Source: CAD feature listing. Evaluate the final solid. Frame: model axes, mm. A direction names the side the tool comes from. Give positions to 0.01 mm unless a question says otherwise; leave off trailing zeros. Order: outer loops, then holes, each group sorted by start corner. A loop starts at its lowest first (then second) coordinate and runs counter-clockwise, first axis right, second up. Notation, with made-up numbers: (28.25, -31) -> (66.25, -31) arc R30 ccw to (66.25, -3) -> close; hole circle Ø11 at (61.5, -23). An arc over 180 degrees is marked (long way). Use CSV: the item, a comma, the result in double quotes.
```python
from build123d import *

# Parameters (mm, degrees)
SKETCH_1_W           = 16
SKETCH_1_H           = 11
EXTRUDE_1_DEPTH      = 25
SKETCH_2_OUTSIDE_W   = 215.706
SKETCH_2_OUTSIDE_H   = 63.306
SKETCH_2_OUTSIDE_R   = 2.15
SKETCH_2_OUTSIDE_R_2 = 6.85
CUT_EXTRUDE_1_DEPTH  = 182.533054841
SKETCH_3_R           = 7.8
CUT_EXTRUDE_2_DEPTH  = 1.3
SKETCH_4_R           = 7.85
CUT_EXTRUDE_3_DEPTH  = 1.3
CUT_EXTRUDE_5_DEPTH  = 7
SKETCH_5_3_R         = 1.50558517
CUT_EXTRUDE_6_DEPTH  = 181.299334441


with BuildPart() as part:
    # 草图1 → 凸台-拉伸1 (new body)
    with BuildSketch(Plane(origin=(0, 0, 0), x_dir=(1, 0, 0), z_dir=(0, 1, 0))):
        Polygon((0, 0), (0, 19), (127, 19), (161, 20.3), (177.4, 20.3), (177.4, 13.4), (146, 13.4), (146, -2.1), (177.4, -2.1), (177.4, -9), (144, -9), (127, 0), align=None)
        with Locations((39, 9.5)):
            Rectangle(SKETCH_1_W, SKETCH_1_H, mode=Mode.SUBTRACT)
        Polygon((126, 15), (126, 4), (143, -5), (143, 15.65), align=None, mode=Mode.SUBTRACT)
        with Locations((58, 9.5)):
            Rectangle(SKETCH_1_W, SKETCH_1_H, mode=Mode.SUBTRACT)
        with Locations((77, 9.5)):
            Rectangle(SKETCH_1_W, SKETCH_1_H, mode=Mode.SUBTRACT)
        with Locations((96, 9.5)):
            Rectangle(SKETCH_1_W, SKETCH_1_H, mode=Mode.SUBTRACT)
        with Locations((115, 9.5)):
            Rectangle(SKETCH_1_W, SKETCH_1_H, mode=Mode.SUBTRACT)
    extrude(amount=EXTRUDE_1_DEPTH)

    # 草图2 outside → 切除-拉伸1 (cut, through all)
    # profile 1 of 3: a face of its own
    with BuildSketch(Plane.XY.offset(9)):
        with Locations((88.7, 12.5)):
            Rectangle(SKETCH_2_OUTSIDE_W, SKETCH_2_OUTSIDE_H)
        Polygon((0, 21.701223904), (3.298776096, 25), (172.796734854, 16.606530291), (177.4, 12.003265146), (177.4, 4.603265146), (172.796734854, 0), (4.701223904, 0), (0, 4.701223904), align=None, mode=Mode.SUBTRACT)
    # profile 2 of 3: a face of its own
    with BuildSketch(Plane.XY.offset(9)):
        with Locations((169.9, 8.303265146)):
            Circle(SKETCH_2_OUTSIDE_R)
    # profile 3 of 3: a face of its own
    with BuildSketch(Plane.XY.offset(9)):
        with Locations((12, 13.201223904)):
            Circle(SKETCH_2_OUTSIDE_R_2)
    extrude(amount=-CUT_EXTRUDE_1_DEPTH, mode=Mode.SUBTRACT)

    # 草图3 → 切除-拉伸2 (cut)
    with BuildSketch(Plane.XY):
        with Locations((12, 13.201223904)):
            Circle(SKETCH_3_R)
    extrude(amount=-CUT_EXTRUDE_2_DEPTH, mode=Mode.SUBTRACT)

    # 草图4 → 切除-拉伸3 (cut)
    with BuildSketch(Plane(origin=(0, 0, -19), x_dir=(-1, 0, 0), z_dir=(0, 0, -1))):
        with Locations((-12, 13.201223904)):
            Circle(SKETCH_4_R)
    extrude(amount=-CUT_EXTRUDE_3_DEPTH, mode=Mode.SUBTRACT)

    # 草图5 → 切除-拉伸5 (cut)
    with BuildSketch(Plane.XY):
        Polygon((15.855153168, 19.304745085), (18.337708884, 17.144440218), (21.449865637, 18.214244102), (22.079466672, 21.444352852), (19.596910956, 23.604657718), (16.484754204, 22.534853834), align=None)
        Polygon((5.896478819, 17.056377072), (8.056783686, 19.538932788), (6.986979802, 22.651089541), (3.756871052, 23.280690576), (1.596566186, 20.79813486), (2.66637007, 17.685978108), align=None)
        Polygon((18.103521181, 9.346070736), (15.943216314, 6.86351502), (17.013020198, 3.751358267), (20.243128948, 3.121757232), (22.403433814, 5.604312948), (21.33362993, 8.7164697), align=None)
        Polygon((8.144846832, 7.097702723), (5.662291116, 9.25800759), (2.550134363, 8.188203706), (1.920533328, 4.958094956), (4.403089044, 2.79779009), (7.515245796, 3.867593974), align=None)
    extrude(amount=-CUT_EXTRUDE_5_DEPTH, mode=Mode.SUBTRACT)

    # 草图5<3> → 切除-拉伸6 (cut, through all)
    with BuildSketch(Plane.XY):
        with Locations((5.03269008, 6.02789884)):
            Circle(SKETCH_5_3_R)
        with Locations((4.826674936, 20.168533824)):
            Circle(SKETCH_5_3_R)
        with Locations((18.96730992, 20.374548968)):
            Circle(SKETCH_5_3_R)
        with Locations((19.173325064, 6.233913984)):
            Circle(SKETCH_5_3_R)
    extrude(amount=-CUT_EXTRUDE_6_DEPTH, mode=Mode.SUBTRACT)


solid = part.part
```
1. Section query C-C on x = 63.5. Return loops of the section in (y, z).
Answer below:
outline,"(0, -19) -> (22.02, -19) -> (22.02, -15) -> (0, -15) -> close; (0, -4) -> (22.02, -4) -> (22.02, 0) -> (0, 0) -> close"
2. Section query A-A on x = 12. Return loops of the section in (y, z), plus the area to 3 significant figures.
Answer below:
outline,"(0, -19) -> (5.35, -19) -> (5.35, -17.7) -> (6.35, -17.7) -> (6.35, -1.3) -> (5.4, -1.3) -> (5.4, 0) -> (0, 0) -> close; (20.05, -17.7) -> (21.05, -17.7) -> (21.05, -19) -> (24.57, -19) -> (24.57, 0) -> (21, 0) -> (21, -1.3) -> (20.05, -1.3) -> close"
area,"201 mm²"
3. Section query D-D on x = 138. Return loops of the section in (y, z), plus the area to 3 significant figures.
Answer below:
outline,"(0, -19.42) -> (18.33, -19.42) -> (18.33, -15.46) -> (0, -15.46) -> close; (0, 2.35) -> (18.33, 2.35) -> (18.33, 5.82) -> (0, 5.82) -> close"
area,"136 mm²"
4. Ray query, line 1 along Z through (x, y) = (54, 6); line 2 along X through (y, z) = (7, -17.25); line 3 along Y through (x, z) = (143.5, -6.75). Return the intervals inside material, ascending.
Answer below:
line 1,"z = -19 to -15, -4 to 0"
line 2,"x = 0 to 3.88, 6.18 to 9.09, 14.91 to 17.88, 20.47 to 168.19, 171.61 to 177.4"
line 3,"y = 0 to 18.06"
5. Mould query, pull axis Z, two halves, no side actions, for faces 6 (the flat face through (20, 22, -7)), 7 (the flat face through (161, 9, 2.1)), 8 (the flat face through (0, 13, -9)), 9 (the flat face through (167, 8, -20.3)). Classes: released by +Z, released by -Z, zero draft, split by the parting line, or undercut.
Answer below:
face 6,"released by +Z"
face 7,"undercut"
face 8,"zero draft"
face 9,"released by -Z"
6. Section query B-B on x = 169.9. Return loops of the section in (y, z), plus the area to 3 significant figures.
Answer below:
outline,"(0, -20.3) -> (6.15, -20.3) -> (6.15, -13.4) -> (0, -13.4) -> close; (0, 2.1) -> (6.15, 2.1) -> (6.15, 9) -> (0, 9) -> close; (10.45, -20.3) -> (16.75, -20.3) -> (16.75, -13.4) -> (10.45, -13.4) -> close; (10.45, 2.1) -> (16.75, 2.1) -> (16.75, 9) -> (10.45, 9) -> close"
area,"172 mm²"
7. Pin query (flat end, axial travel): P1, Ø7, axis at x = 5, y = 19, coming from the +Z side; P2, Ø10, axis at x = 58.5, y = 17.5, coming from the -Z side; P3, Ø1.5, axis at x = 159, y = 10.5, coming from the -Z side; P4, Ø9.5, axis at x = 12, y = 13.2, coming from the -Z side. Return the tip coordinate at first contact, or that it passes through.
Answer below:
P1,"stops at z = 0"
P2,"stops at z = -19"
P3,"stops at z = -20.25"
P4,"passes through"
8. Access query for faces 1 (the flat face through (21.876, 7.139, -3.451)), 2 (the flat face through (63, 10, -19)), 3 (the flat face through (146, 9, -6)), 4 (the flat face through (50, 11, -9)), 5 (the flat face through (175.131, 2.334, 5.598)). Directions: +Z, -Z, +X, -X, +Y, -Y. A direction counts if a zero-diameter tool reaches every point of the face in a straight line with its end or side. Return the directions, or none.
Answer below:
face 1,"+Z"
face 2,"-Z, -X, +Y, -Y"
face 3,"+X, +Y, -Y"
face 4,"+Y, -Y"
face 5,"+Z, -Z, +X, -Y"
